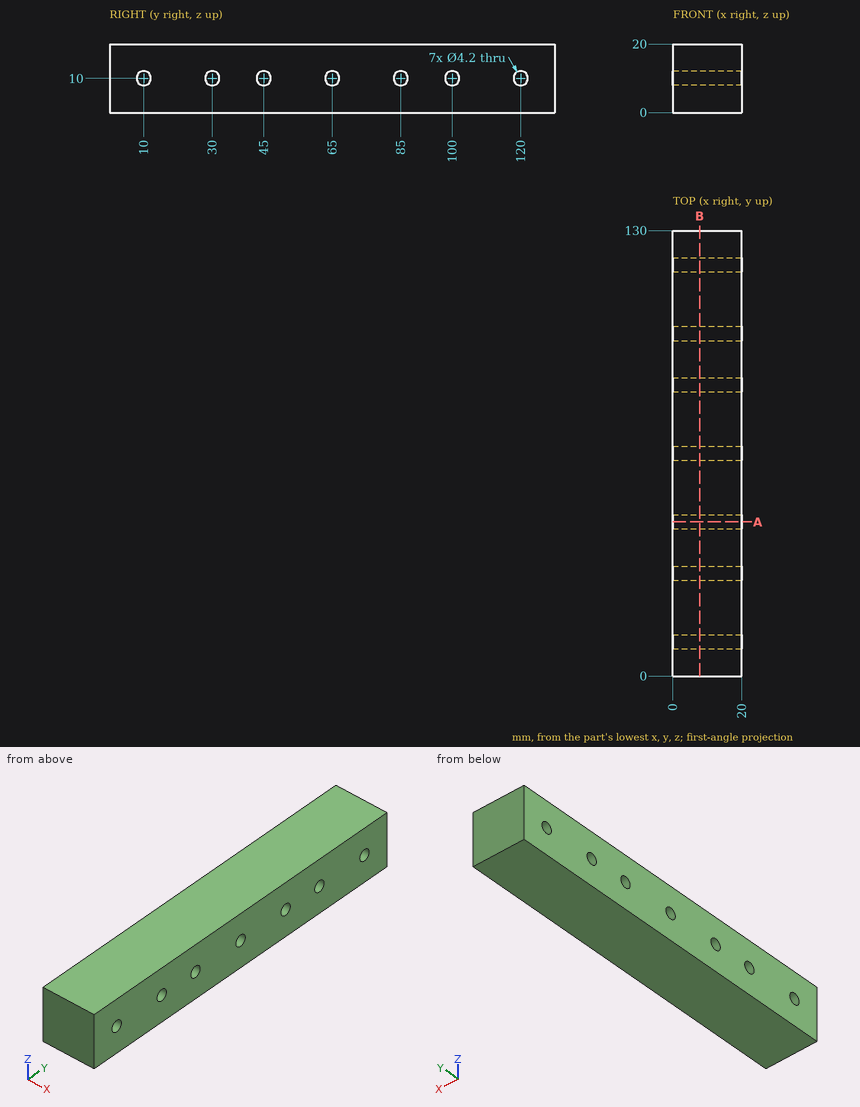
Study the drawing (mm; zero at the part's minimum x, y, z) and answer. Round coordinates to 2 decimals unless told otherwise and drop trailing zeros. Order: outer loops, then holes, each group sorted by start corner. A loop starts at its lowest first (then second) coordinate and runs counter-clockwise, first axis right, second up. Notation, with made-up numbers: (-24, -13) - (-18, -13) arc R23 ccw to (-18, 4) - close; hole circle Ø2 at (81, 37.25). An arc over 180 degrees is marked (long way). Use one line per item in the form item = value. Start each with the question number.
(1) Flat-ended cylindrical pins translate along their axes: pin 1 Ø1 at (y, z) = (100, 13.5) entering from -X; pin 2 Ø4 at (y, z) = (85, 10) entering from -X. Find the tip coordinate at first contact, or state that the pin passes through.
(2) The part is cut by section A-A (y = 45). Give the vertices of the cut face in (x, z), then the cut area to 3 significant figures.
(3) The part is cut by section B-B (x = 7.75). Give the vertices of the cut face in (y, z).
(4) Find the intervals of material crossed by line 1 along Z through (x, y) = (8.5, 120), in increasing order. Write a range as from..to.
Checked values:
q1.pin_1 = 0
q1.pin_2 = through
q2.outline = (0, 0) - (20, 0) - (20, 7.9) - (0, 7.9) - close; (0, 12.1) - (20, 12.1) - (20, 20) - (0, 20) - close
q2.area = 316 mm^2
q3.outline = (0, 0) - (130, 0) - (130, 20) - (0, 20) - close; hole circle Ø4.2 at (10, 10); hole circle Ø4.2 at (30, 10); hole circle Ø4.2 at (45, 10); hole circle Ø4.2 at (65, 10); hole circle Ø4.2 at (85, 10); hole circle Ø4.2 at (100, 10); hole circle Ø4.2 at (120, 10)
q4.line_1 = 0..7.9, 12.1..20
